Design review of the part built by this model. Coordinates are the model's own, in mm. Face numbers are marked on the shaded views. Give positions to 0.01 mm unless a question says otherwise; leave off trailing zeros. Order: outer loops, then holes, each group sorted by start corner. A loop starts at its lowest first (then second) coordinate and runs counter-clockwise, first axis right, second up. Notation, with made-up numbers: (-24, 70) -> (24, 70) arc R16 cw to (24, 76) -> close; hole circle Ø6 at (80, 46). An arc over 180 degrees is marked (long way). One line per item, written item: value. Start each with the question number.
1) For pin 1 (1.4 mm diameter, centred on x = 123, z = -48, fed in from +Y); pin 2 (2.5 mm diameter, centred on x = 98, y = -5, fed in from -Z); pin 3 (3 mm diameter, centred on x = 61, z = 0.5, fed in from -Y); pin 4 (7.5 mm diameter, centred on y = 0, z = 38.1, fed in from -X), all flat-tipped, find the tip position at first contact; note any pin that passes through.
2) Consider section D-D (y = -3.5). State the section outline as (x, z) points.
3) Consider section B-B (x = 139). State how many separate pieces and enclosed holes the cut face has, plus the area to 3 significant figures.
4) The part is to be moulded in two halves that separate along X. For the marked faces 1, 2, 3 and 4, say which applies: released by +X, released by -X, zero draft, split by the parting line, or undercut.
5) Wall thickness on line 1 along X through (y, z) = (-22.5, 36); line 2 along Z through (x, y) = (109.5, -1); line 3 along Z through (x, y) = (174, -7): over which ranges is each line inside the solid? List them lowest first. Write a range as from..to.
6) Consider section C-C (z = 11.5). State the section outline as (x, y) points, plus the area to 3 significant figures.
7) Consider section A-A (y = -23). State the section outline as (x, z) points.
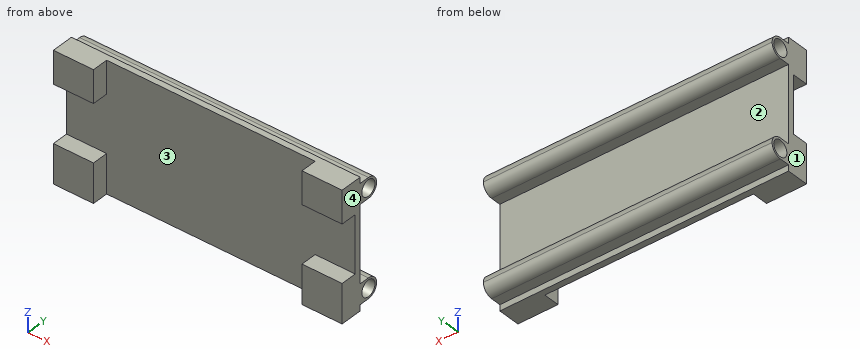
from build123d import *

# Parameters (mm, degrees)
F0_R     = 6.35
F1_DEPTH = 228.6
F2_W     = 165.1
F2_H     = 25.7380759895
F2_H_2   = 10.3431178749
F2_H_3   = 45.0917202979
F2_H_4   = 30.7702037126
F2_H_5   = 15.0568821251
F2_W_2   = 31.75
F3_DEPTH = 12.7


with BuildPart() as f1:
    # F0 (on Right) → F1 (new body)
    with BuildSketch(Plane.YZ):
        with BuildLine():
            ThreePointArc((0, 30.1625), (-7.9375, 38.1), (0, 46.0375))
            Line((0, 46.0375), (-7.9375, 46.0375))
            Line((-7.9375, 46.0375), (-7.9375, 50.8))
            Line((-7.9375, 50.8), (-25.4, 50.8))
            Line((-25.4, 50.8), (-25.4, -50.8))
            Line((-25.4, -50.8), (-7.9375, -50.8))
            Line((-7.9375, -50.8), (-7.9375, -46.0375))
            Line((-7.9375, -46.0375), (0, -46.0375))
            ThreePointArc((0, -46.0375), (-7.9375, -38.1), (0, -30.1625))
            Line((0, -30.1625), (-7.9375, -30.1625))
            Line((-7.9375, -30.1625), (-7.9375, 30.1625))
            Line((-7.9375, 30.1625), (0, 30.1625))
        make_face()
        with BuildLine():
            ThreePointArc((7.9375, -38.1), (5.6126600757, -32.4873399243), (0, -30.1625))
            ThreePointArc((0, -30.1625), (-7.9375, -38.1), (0, -46.0375))
            ThreePointArc((0, -46.0375), (5.6126600757, -43.7126600757), (7.9375, -38.1))
        make_face()
        with Locations((0, -38.1)):
            Circle(F0_R, mode=Mode.SUBTRACT)
        with BuildLine():
            ThreePointArc((0, 30.1625), (5.6126600757, 32.4873399243), (7.9375, 38.1))
            ThreePointArc((7.9375, 38.1), (5.6126600757, 43.7126600757), (0, 46.0375))
            ThreePointArc((0, 46.0375), (-7.9375, 38.1), (0, 30.1625))
        make_face()
        with Locations((0, 38.1)):
            Circle(F0_R, mode=Mode.SUBTRACT)
    extrude(amount=F1_DEPTH)

    # F2 (on face) → F3 (cut)
    with BuildSketch(Plane.XZ.offset(25.4)):
        with Locations((114.3, 37.9309620053)):
            Rectangle(F2_W, F2_H)
        with Locations((114.3, 55.9715589374)):
            Rectangle(F2_W, F2_H_2)
        with Locations((114.3, 2.5160638615)):
            Rectangle(F2_W, F2_H_3)
        with Locations((114.3, -35.4148981437)):
            Rectangle(F2_W, F2_H_4)
        with Locations((114.3, -58.3284410626)):
            Rectangle(F2_W, F2_H_5)
        with Locations((15.875, 2.5160638615)):
            Rectangle(F2_W_2, F2_H_3)
        with Locations((212.725, 2.5160638615)):
            Rectangle(F2_W_2, F2_H_3)
    extrude(amount=-F3_DEPTH, mode=Mode.SUBTRACT)


solid = f1.part
Checked values:
1. pin 1: stops at y = -7.94
1. pin 2: stops at z = -46.04
1. pin 3: stops at y = -12.7
1. pin 4: passes through
2. outline: (0, -46.04) -> (228.6, -46.04) -> (228.6, -43.4) -> (0, -43.4) -> close; (0, -32.8) -> (228.6, -32.8) -> (228.6, -30.16) -> (0, -30.16) -> close; (0, 30.16) -> (228.6, 30.16) -> (228.6, 32.8) -> (0, 32.8) -> close; (0, 43.4) -> (228.6, 43.4) -> (228.6, 46.04) -> (0, 46.04) -> close
3. separate pieces: 1
3. enclosed holes: 2
3. area: 680 mm^2
4. face 1: released by -X
4. face 2: zero draft
4. face 3: undercut
4. face 4: released by +X
5. line 1: x = 0..31.75, 196.85..228.6
5. line 2: z = -46.04..-44.37, -31.83..-30.16, 30.16..31.83, 44.37..46.04
5. line 3: z = -46.04..-30.16, 30.16..46.04
6. outline: (0, -12.7) -> (228.6, -12.7) -> (228.6, -7.94) -> (0, -7.94) -> close
6. area: 1,090 mm^2
7. outline: (0, -50.8) -> (31.75, -50.8) -> (31.75, -20.03) -> (0, -20.03) -> close; (0, 25.06) -> (31.75, 25.06) -> (31.75, 50.8) -> (0, 50.8) -> close; (196.85, -50.8) -> (228.6, -50.8) -> (228.6, -20.03) -> (196.85, -20.03) -> close; (196.85, 25.06) -> (228.6, 25.06) -> (228.6, 50.8) -> (196.85, 50.8) -> close
